CAD build for the part. Positions are in the model's coordinates, mm. A direction names the side the tool comes from. Give positions to 0.01 mm unless a question says otherwise; leave off trailing zeros. Loops run counter-clockwise (first coordinate to the right, second up) from the corner with the lowest first, then second, coordinate; pieces in that order, holes last.
```python
from build123d import *

# Parameters (mm, degrees)
F0_W     = 381
F0_H     = 69.85
F1_DEPTH = 15.875
F2_W     = 6.35
F2_H     = 6.604
F3_DEPTH = 381


with BuildPart() as f1:
    # F0 (on Right) → F1 (new body)
    with BuildSketch(Plane.YZ):
        with Locations((190.5, 34.925)):
            Rectangle(F0_W, F0_H)
    extrude(amount=F1_DEPTH)

    # F2 (on face) → F3 (cut, through all)
    with BuildSketch(Plane.XZ):
        with Locations((12.7, 6.477)):
            Rectangle(F2_W, F2_H)
    extrude(amount=-F3_DEPTH, mode=Mode.SUBTRACT)


solid = f1.part
```
1. Saw through at A-A, the plane y = 35.5. List the corners of the cut face in (x, z) (3 decimals), and give its area (3 significant figures).
Responses:
outline: (0, 0) - (15.875, 0) - (15.875, 3.175) - (9.525, 3.175) - (9.525, 9.779) - (15.875, 9.779) - (15.875, 69.85) - (0, 69.85) - close
area: 1,070 mm2
2. Pull direction Z, two halves, no side cores. Call faces 1 (the face through (0, 188, 35)), 2 (the face through (9.525, 188, 6)), 3 (the face through (8, 188, 0)): released by +Z, released by -Z, zero draft, split by the parting line, or undercut.
Responses:
face 1: zero draft
face 2: undercut
face 3: released by -Z
3. Probe line 1 along Z through (x, y) = (14, 195.5) (3 decimals); line 2 along X through (y, z) = (311.5, 5) (3 decimals). List the from-to ranges inside material, lowest first.
Responses:
line 1: z = 0 to 3.175, 9.779 to 69.85
line 2: x = 0 to 9.525
4. Tool access for faces 4 (the face through (15.875, 188, 40)), 5 (the face through (13, 188, 3.175)): list every direction of +Z, -Z, +X, -X, +Y, -Y with a clear straight run to the whole face (end or side of a thin tool).
Responses:
face 4: +Z, -Z, +X, +Y, -Y
face 5: +X, +Y, -Y
5. Drop a flat-ended pin along its axis: pin 1 (3.5 mm diameter, centred on y = 240, z = 7.5, fed in from +X) (3 decimals). Give the stop position or say it passes through.
Responses:
pin 1: stops at x = 9.525
